Design review of the part built by this model. Coordinates are the model's own, in mm. Coordinates: 2 decimals unless noted, no trailing zeros. Loops run counter-clockwise (first coordinate to the right, second up) from the corner with the lowest first, then second, coordinate; pieces in that order, holes last. Notation, with made-up numbers: (52.25, -14) -> (108.25, -14) arc R22 cw to (108.25, -2) -> close; hole circle Ø9 at (-11, 18). An arc over 180 degrees is marked (long way). Use a Markdown table: item, result. Add a question column.
Q1. Take a section at A-A on x = 0. Write out the cut boundary in (y, z), plus the area to 3 significant figures.
Q2. For probe 1 along Y at (x, z) = (0, -5.5); probe 2 along Y at (x, z) = (-0.5, 34); probe 3 along X at (y, z) = (1.5, -10.5), list the stretches that pass through material, from the lowest coordinate up.
Q3. Clearance check with flat-ended pins moving along their axes: pin 1 Ø1.5 at (y, z) = (5, 3) entering from -X; pin 2 Ø2 at (x, z) = (-2.5, -15.5) entering from -Y; pin 3 Ø6 at (x, z) = (5.5, -18.5) entering from +Y. State where each tip first meets the part, or that it passes through.
Q4. Take a section at C-C on z = -29. Write out the cut boundary in (x, y), plus the area to 3 significant figures.
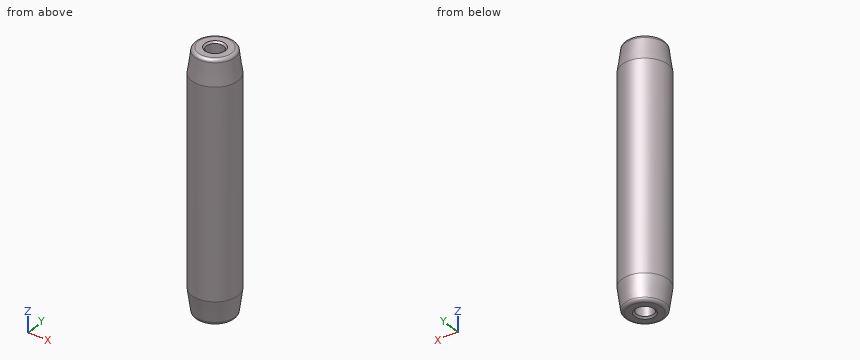
from build123d import *

# Parameters (mm, degrees)
F2_R    = 1
F3_SIZE = 0.5


with BuildPart() as f1:
    # F0 (on Front) → F1 (revolve)
    with BuildSketch(Plane.XZ):
        Polygon((5.75, 37.5), (2.5, 37.5), (2.5, -37.5), (5.75, -37.5), (6.75, -30.3), (6.75, 30.3), align=None)
    revolve(axis=Axis((0, 0, 0), (0, 0, 1)))

    # F2
    f2_edges = [f1.edges().sort_by_distance(p)[0] for p in [
        (-5.75, 0, 37.5),
        (-5.75, 0, -37.5),
    ]]
    fillet(f2_edges, radius=F2_R)

    # F3
    f3_edges = [f1.edges().sort_by_distance(p)[0] for p in [
        (-2.5, 0, 37.5),
        (-2.5, 0, -37.5),
    ]]
    chamfer(f3_edges, length=F3_SIZE)


solid = f1.part
Answer list:
| question | item | result |
|---|---|---|
| 1 | outline | (-6.75, -30.3) -> (-5.87, -36.64) arc R1 ccw to (-4.88, -37.5) -> (-3, -37.5) -> (-2.5, -37) -> (-2.5, 37) -> (-3, 37.5) -> (-4.88, 37.5) arc R1 ccw to (-5.87, 36.64) -> (-6.75, 30.3) -> close; (2.5, -37) -> (3, -37.5) -> (4.88, -37.5) arc R1 ccw to (5.87, -36.64) -> (6.75, -30.3) -> (6.75, 30.3) -> (5.87, 36.64) arc R1 ccw to (4.88, 37.5) -> (3, 37.5) -> (2.5, 37) -> close |
| 1 | area | 622 mm² |
| 2 | probe 1 | -6.75 to -2.5, 2.5 to 6.75 |
| 2 | probe 2 | -6.22 to -2.45, 2.45 to 6.22 |
| 2 | probe 3 | -6.58 to -2, 2 to 6.58 |
| 3 | pin 1 | x = -5.24 |
| 3 | pin 2 | y = -6.58 |
| 3 | pin 3 | y = 6.27 |
| 4 | outline | circle Ø13.5 at (0, 0); hole circle Ø5 at (0, 0) |
| 4 | area | 124 mm² |
